from build123d import *

# Parameters (mm, degrees)
EXTRUDE_2_DEPTH     = 19.5
SKETCH_3_R          = 2
EXTRUDE_3_DEPTH     = 1.5
SKETCH_4_W          = 9.8
SKETCH_4_H          = 5.9
EXTRUDE_4_DEPTH     = 0.5
SKETCH_4_3_W        = 9.8
SKETCH_4_3_H        = 5.9
EXTRUDE_5_DEPTH     = 8
CUT_EXTRUDE_1_DEPTH = 23.835608234
SKETCH_7_R          = 1.5
CUT_EXTRUDE_2_DEPTH = 25.167333429
FILLET_1_R          = 0.2
SKETCH_8_W          = 2
SKETCH_8_H          = 5.9
EXTRUDE_6_DEPTH     = 2
CHAMFER_1_SIZE2     = 2
CHAMFER_1_SIZE      = 1.154700538
FILLET_2_R          = 0.5
CHAMFER_2_SIZE      = 0.5


with BuildPart() as part:
    # 스케치2 → 보스-돌출2 (new body)
    with BuildSketch(Plane.XY):
        with BuildLine():
            Line((-7.455870171, 2.9), (-9.308732459, 2.9))
            ThreePointArc((-9.308732459, 2.9), (-9.749858874, -0.052458871), (-9.276987658, -3))
            Line((-9.276987658, -3), (-7.416198487, -3))
            ThreePointArc((-7.416198487, -3), (-7.999819157, -0.053790897), (-7.455870171, 2.9))
        make_face()
    extrude(amount=EXTRUDE_2_DEPTH)

    # 스케치3 → 보스-돌출3 (add)
    with BuildSketch(Plane(origin=(-8, 0, 0), x_dir=(0, 0, -1), z_dir=(1, 0, 0))):
        with Locations(Location((-3.25, 0, 0), (0, 0, 180))):
            Circle(SKETCH_3_R)
    extrude(amount=EXTRUDE_3_DEPTH)

    # 스케치4 → 보스-돌출4 (add, symmetric)
    with BuildSketch(Plane.ZY.offset(9.75)):
        with Locations((9.15, -0.05)):
            Rectangle(SKETCH_4_W, SKETCH_4_H)
    extrude(amount=EXTRUDE_4_DEPTH, both=True)

    # 스케치4<3> → 보스-돌출5 (add)
    with BuildSketch(Plane.ZY.offset(9.75)):
        with Locations((9.15, -0.05)):
            Rectangle(SKETCH_4_3_W, SKETCH_4_3_H)
    extrude(amount=EXTRUDE_5_DEPTH)

    # 스케치6 → 컷-돌출1 (cut, through all)
    with BuildSketch(Plane.XY.offset(14.05)):
        with BuildLine():
            Line((-12.672410978, 2.9), (-17.75, 2.9))
            Line((-17.75, 2.9), (-17.75, -3))
            Line((-17.75, -3), (-12.649110641, -3))
            ThreePointArc((-12.649110641, -3), (-12.999898626, -0.051339326), (-12.672410978, 2.9))
        make_face()
    extrude(amount=-CUT_EXTRUDE_1_DEPTH, mode=Mode.SUBTRACT)

    # 스케치7 → 컷-돌출2 (cut, through all)
    with BuildSketch(Plane(origin=(0, 2.9, 0), x_dir=(1, 0, 0), z_dir=(0, 1, 0))):
        with Locations(Location((-9.955870171, -9.25, 0), (0, 0, 180))):
            Circle(SKETCH_7_R)
    extrude(amount=-CUT_EXTRUDE_2_DEPTH, mode=Mode.SUBTRACT)

    # 필렛1
    fillet_1_edges = [part.edges().sort_by_distance(p)[0] for p in [
        (-8.455870171, -3, 9.25),
        (-8.455870171, 2.9, 9.25),
    ]]
    fillet(fillet_1_edges, radius=FILLET_1_R)

    # 스케치8 → 보스-돌출6 (add)
    with BuildSketch(Plane(origin=(-8, 0, 0), x_dir=(0, 0, -1), z_dir=(1, 0, 0))):
        with Locations((-18.5, -0.05)):
            Rectangle(SKETCH_8_W, SKETCH_8_H)
    extrude(amount=EXTRUDE_6_DEPTH)

    # 모따기1
    chamfer_1_edges = [part.edges().sort_by_distance(p)[0] for p in [
        (-6, -0.05, 19.5),
    ]]
    chamfer_1_side = [part.faces().sort_by_distance(p)[0] for p in [
        (-6.023094011, -0.05, 19.5),
    ]]
    chamfer(chamfer_1_edges, length=CHAMFER_1_SIZE - 0.0001, length2=CHAMFER_1_SIZE2 - 0.0001, reference=chamfer_1_side[0])  # a hair under: the kernel refuses the full size

    # 필렛2
    fillet_2_edges = [part.edges().sort_by_distance(p)[0] for p in [
        (-7.999819157, -0.053790897, 17.5),
    ]]
    fillet(fillet_2_edges, radius=FILLET_2_R)

    # 모따기2
    chamfer_2_edges = [part.edges().sort_by_distance(p)[0] for p in [
        (-9.749858874, -0.052458871, 0),
        (-12.999898626, -0.051339326, 4.25),
        (-12.999898626, -0.051339326, 14.05),
        (-9.749858874, -0.052458871, 19.5),
    ]]
    chamfer(chamfer_2_edges, length=CHAMFER_2_SIZE)


solid = part.part
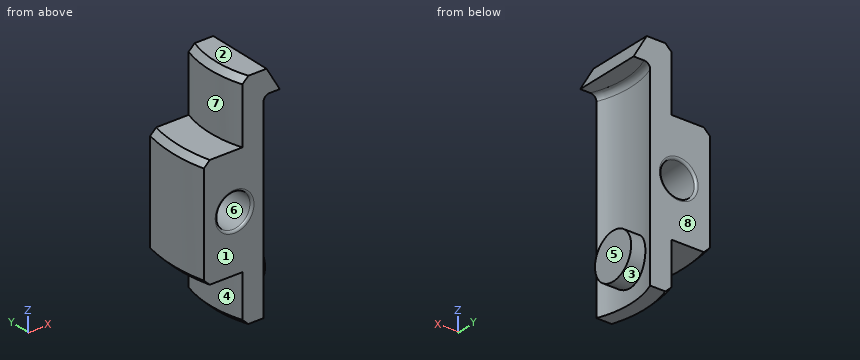
Work out the finished part from the listing and answer in its coordinate system (mm). Face numbers are marked on the shaded views. A direction names the side the tool comes from. Coordinates: 2 decimals unless noted, no trailing zeros. Loops run counter-clockwise (first coordinate to the right, second up) from the corner with the lowest first, then second, coordinate; pieces in that order, holes last. Notation, with made-up numbers: (64.5, 65) -> (102.5, 65) arc R23 cw to (102.5, 103) -> close; hole circle Ø3 at (28.25, 35.5). An arc over 180 degrees is marked (long way). Write each question's results on one line, items separated by ' | '. Start each with the question number.
1) For the marked faces 4, 5, 6, 7 and 8, determine the directions among +Z, -Z, +X, -X, +Y, -Y from which every point of the face is accessible in a straight line to the end or side of a thin tool.
2) Find section C-C on z = 13. Determine the outline of the cut face in (x, y), then the cut area to 3 significant figures.
3) Find section A-A on z = 3.25. Determine the outline of the cut face in (x, y), then the cut area to 3 significant figures.
4) The mould has two halves that part along Z. Classify the marked faces 1, 2 and 3: pulls with the +Z half, pulls with the -Z half, needs draft (parallel to the pull), parting line crosses it, or undercut.
5) Find section B-B on x = -6.25. Determine the outline of the cut face in (y, z), then the cut area to 3 significant figures.
6) Consider line 1 along Z through (x, y) = (-12, -1.9); line 2 along X through (y, z) = (2.6, 9); line 3 along Z through (x, y) = (-7, -0.7). Determine where each line is inside the solid, lowest interval first.
7) Flat-ended cylindrical pins translate along their axes: P1, Ø2, axis at x = -11.5, y = -0.5, coming from the +Z side; P2, Ø1.2, axis at x = -7, y = 1, coming from the -Z side; P3, Ø3, axis at x = -8.5, y = 1.5, coming from the -Z side; P4, Ø1, axis at x = -11.5, y = 0.5, coming from the -Z side. Find the tip coordinate at first contact, or state that the pin passes through.
Response values:
1) face 4: -Z, -X | face 5: -Z, +X, +Y, -Y | face 6: +Y, -Y | face 7: +Z, -X | face 8: +Z, -Z, +X, -X, +Y
2) outline: (-12.67, 2.9) arc R13 ccw to (-12.65, -3) -> (-7.42, -3) arc R8 cw to (-7.46, 2.9) -> close | area: 29.9 mm^2
3) outline: (-9.31, 2.9) arc R9.75 ccw to (-9.28, -3) -> (-7.42, -3) arc R8 cw to (-7.75, -2) -> (-6.5, -2) -> (-6.5, 2) -> (-7.75, 2) arc R8 cw to (-7.46, 2.9) -> close | area: 16.2 mm^2
4) face 1: needs draft | face 2: pulls with the +Z half | face 3: undercut
5) outline: (-3, 17.5) -> (2.9, 17.5) -> (2.9, 17.93) -> (-3, 17.93) -> close | area: 2.56 mm^2
6) line 1: z = 4.25 to 14.05 | line 2: x = -12.74 to -11.43, -8.48 to -7.57 | line 3: z = 1.38 to 5.12, 17.5 to 19.23
7) P1: stops at z = 14.05 | P2: stops at z = 1.29 | P3: stops at z = 0 | P4: stops at z = 4.25
